Could you check a few things on this drawing? It's one solid part, dimensions in mm from its lowest x, y, z. A direction names the side the tool comes from. Round coordinates to 2 decimals unless told otherwise and drop trailing zeros. Write each loop counter-clockwise with the first axis right and the second up, starting at its lowest first coordinate (ties: lowest second). Pieces come first, ordered by that corner, then holes. Notation, with made-up numbers: M 17,1.25 L 74,1.25 A11 ccw 74,13.25 Z; hole C 68,87 d1. An arc over 180 degrees is marked long. One line per question, with ' | ' between items. Start each with the question number.
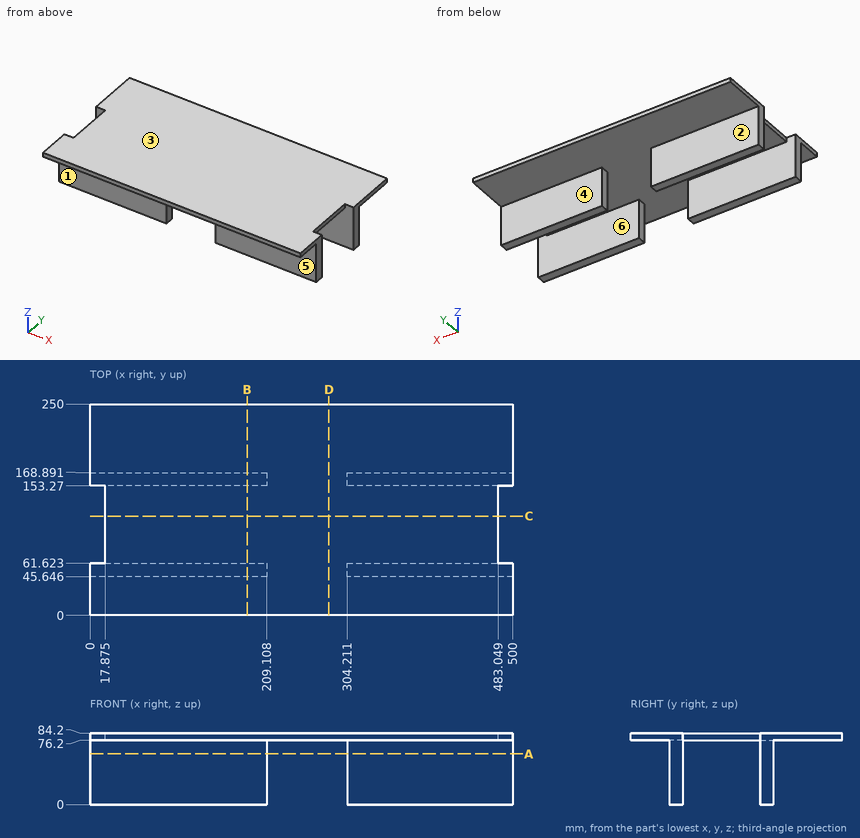
1. Suppose I cut it at B-B (x = 186). Write out the boundary of the cut face in (y, z) (1 decimal).
2. Which directions (+Z, -Z, +X, -X, +Y, -Y) give clear straight access to the entire face, cutting with the end or side of a thin tool? Please do the marked faces 1, 2 and 3.
3. I'm going to push flat-ended pins straight in: P1, Ø23, axis at x = 377, z = 26.5, coming from the -Y side; P2, Ø6.5, axis at y = 123.5, z = 79, coming from the -X side (1 decimal); P3, Ø10, axis at x = 430, z = 10, coming from the +Y side. Where does each tip first touch, or does it pass through?
4. Suppose I cut it at A-A (z = 60). Write out the boundary of the cut face in (x, y) (1 decimal), and give its area (3 significant figures).
5. I need wall thicknesses on line 1 along Y through (x, z) = (115.5, 75.5) (1 decimal); line 2 along X through (y, z) = (156, 55); line 3 along Z through (x, y) = (248, 130). Which ranges of each line are inside material? Lowest first, please. Write a range as from..to.
6. Suppose I cut it at D-D (x = 282.5). Write out the boundary of the cut face in (y, z), and give its area (3 significant figures).
7. Suppose I cut it at C-C (y = 117.5). Write out the boundary of the cut face in (x, z) (1 decimal).
8. If we mould it in two halves opening along Y, with no side actions, what happens to the marked faces 4, 5 and 6? For each: released by +Y, released by -Y, zero draft, split by the parting line, or undercut.
Computed:
1) outline: M 0,76.2 L 45.6,76.2 L 45.6,0 L 61.6,0 L 61.6,76.2 L 153.3,76.2 L 153.3,0 L 168.9,0 L 168.9,76.2 L 250,76.2 L 250,84.2 L 0,84.2 Z
2) face 1: -Z, +X, -X, -Y | face 2: -Z, +X, -X, +Y | face 3: +Z, +X, -X, +Y, -Y
3) P1: stops at y = 45.65 | P2: stops at x = 17.9 | P3: stops at y = 168.89
4) outline: M 0,45.6 L 209.1,45.6 L 209.1,61.6 L 0,61.6 Z; M 0,153.3 L 209.1,153.3 L 209.1,168.9 L 0,168.9 Z; M 304.2,45.6 L 500,45.6 L 500,61.6 L 304.2,61.6 Z; M 304.2,153.3 L 500,153.3 L 500,168.9 L 304.2,168.9 Z | area: 12,800 mm²
5) line 1: y = 45.6..61.6, 153.3..168.9 | line 2: x = 0..209.11, 304.21..500 | line 3: z = 76.2..84.2
6) outline: M 0,76.2 L 250,76.2 L 250,84.2 L 0,84.2 Z | area: 2,000 mm²
7) outline: M 17.9,76.2 L 483,76.2 L 483,84.2 L 17.9,84.2 Z
8) face 4: released by +Y | face 5: released by -Y | face 6: undercut
